from build123d import *

# Parameters (mm, degrees)
SKETCH1_R                                 = 7.9375
SKETCH1_R_2                               = 3.2639
SKETCH1_R_3                               = 1.575
INNER_SIDE_EXTRUDE_DEPTH                  = 2.032
OUTER_START                               = -9.525
SKETCH1_3_R                               = 7.9375
SKETCH1_3_R_2                             = 1.575
SKETCH1_3_R_3                             = 3.2639
OUTER_SIDE_EXTRUDE_DEPTH                  = 9.525
CLEVIS_PIN_CUT_DEPTH                      = 15.721869362
CLEVIS_PIN_CUT_DEPTH_BACK                 = 15.721869362
SKETCH2_R                                 = 1.63195
CHAMFER_SO_STEVE_DOESN_T_CUT_HIMSELF_SIZE = 0.396875
CUT_EXTRUDE1_DEPTH                        = 15.72186947
CUT_EXTRUDE1_DEPTH_BACK                   = 15.72186947
SKETCH4_W                                 = 19.05
SKETCH4_H                                 = 4.803702905


with BuildPart() as part:
    # Sketch1 → Inner Side Extrude (new body)
    with BuildSketch(Plane(origin=(0, 0, 0), x_dir=(0, 0, -1), z_dir=(1, 0, 0))):
        Circle(SKETCH1_R)
        Circle(SKETCH1_R_2, mode=Mode.SUBTRACT)
        with Locations((-5.588, 0)):
            Circle(SKETCH1_R_3, mode=Mode.SUBTRACT)
        with Locations((5.588, 0)):
            Circle(SKETCH1_R_3, mode=Mode.SUBTRACT)
    extrude(amount=INNER_SIDE_EXTRUDE_DEPTH)

    # Sketch1_3 → Outer Side Extrude (add)
    with BuildSketch(Plane(origin=(0, 0, 0), x_dir=(0, 0, -1), z_dir=(1, 0, 0)).offset(OUTER_START)):
        Circle(SKETCH1_3_R)
        with Locations((5.588, 0)):
            Circle(SKETCH1_3_R_2, mode=Mode.SUBTRACT)
        with Locations((-5.588, 0)):
            Circle(SKETCH1_3_R_2, mode=Mode.SUBTRACT)
        Circle(SKETCH1_3_R_3, mode=Mode.SUBTRACT)
    extrude(amount=OUTER_SIDE_EXTRUDE_DEPTH)

    # Sketch2 → Clevis Pin Cut (cut, two sides: drawn at the far end of the back side and taken through both)
    with BuildSketch(Plane(origin=(0, 0, 0), x_dir=(1, 0, 0), z_dir=(0, 1, 0)).offset(-CLEVIS_PIN_CUT_DEPTH_BACK)):
        with Locations(Location((-3.1242, 0, 0), (0, 0, 270))):
            Circle(SKETCH2_R)
    extrude(amount=CLEVIS_PIN_CUT_DEPTH + CLEVIS_PIN_CUT_DEPTH_BACK, mode=Mode.SUBTRACT)

    # Chamfer so Steve Doesn_t cut himself
    chamfer_so_steve_doesn_t_cut_himself_edges = [part.edges().sort_by_distance(p)[0] for p in [
        (2.032, 0, 3.2639),
        (-9.525, 0, 7.9375),
        (-9.525, 0, 3.2639),
    ]]
    chamfer(chamfer_so_steve_doesn_t_cut_himself_edges, length=CHAMFER_SO_STEVE_DOESN_T_CUT_HIMSELF_SIZE)

    # Sketch4 → Cut-Extrude1 (cut, two sides: drawn at the far end of the back side and taken through both)
    with BuildSketch(Plane.XY.offset(-CUT_EXTRUDE1_DEPTH_BACK)):
        with Locations((-3.1242, -7.481851452)):
            Rectangle(SKETCH4_W, SKETCH4_H)
        with Locations((-3.1242, 7.481851452)):
            Rectangle(SKETCH4_W, SKETCH4_H)
    extrude(amount=CUT_EXTRUDE1_DEPTH + CUT_EXTRUDE1_DEPTH_BACK, mode=Mode.SUBTRACT)


solid = part.part
Check sheet for the modelled part. Datum: model origin and axes. Units: mm. Round coordinates to 2 decimals unless told otherwise and drop trailing zeros. Order: outer loops, then holes, each group sorted by start corner. A loop starts at its lowest first (then second) coordinate and runs counter-clockwise, first axis right, second up.
(1) Cross-section at B-B, the plane z = 0. Enter the section's corners in (x, y) (3 decimals), and give its area (3 significant figures).
(2) Scan lines: probe 1 along X at (y, z) = (-4.55, 0) (3 decimals); probe 2 along Y at (x, z) = (-4.25, -3); probe 3 along Y at (x, z) = (-4.75, 5.5). Record each from-to range of solid material in increasing order.
(3) Draft check along Z on faces 1 (the flat face through (-9.525, 3.5, 1.8)), 2 (the cylindrical face through (-2.634, -3.969, 1.557)), 3 (the cylindrical face through (-3.626, -0.077, -7.937)), 4 (the cylindrical face through (-2.634, 3.937, 1.557)). Enter one of: pulls with the +Z half, pulls with the -Z half, needs draft (parallel to the pull), parting line crosses it, or undercut.
(4) Cross-section at A-A, the plane y = 0. State how many separate pieces and enclosed holes the cut face has, and give its area (3 significant figures).
Check sheet entries:
1. outline: (-9.525, -5.08) - (-4.756, -5.08) - (-4.756, -3.264) - (-9.128, -3.264) - (-9.525, -3.661) - close; (-9.525, 3.661) - (-9.128, 3.264) - (-4.756, 3.264) - (-4.756, 5.08) - (-9.525, 5.08) - close; (-1.492, -5.08) - (2.032, -5.08) - (2.032, -3.661) - (1.635, -3.264) - (-1.492, -3.264) - close; (-1.492, 3.264) - (1.635, 3.264) - (2.032, 3.661) - (2.032, 5.08) - (-1.492, 5.08) - close
1. area: 29.8 mm2
2. probe 1: x = -9.525 to -4.756, -1.492 to 2.032
2. probe 2: y = -5.08 to -1.29, 1.29 to 5.08
2. probe 3: y = -5.08 to -1.57, 1.57 to 5.08
3. face 1: needs draft
3. face 2: undercut
3. face 3: pulls with the -Z half
3. face 4: undercut
4. separate pieces: 4
4. enclosed holes: 0
4. area: 34.7 mm2
